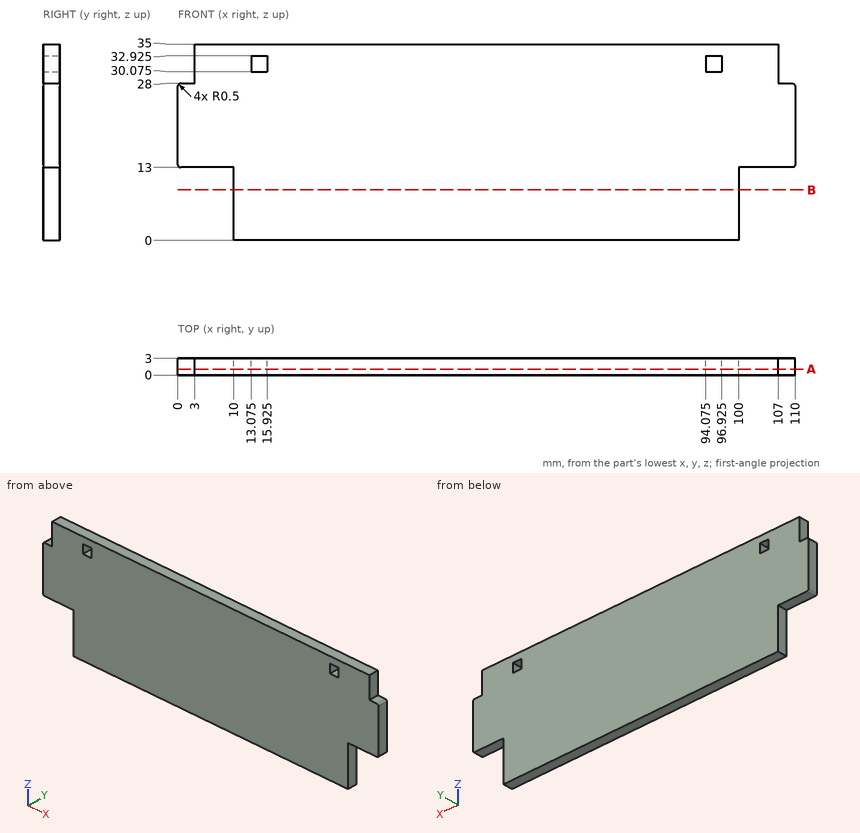
Study the drawing (mm; zero at the part's minimum x, y, z) and answer. Coordinates: 2 decimals unless noted, no trailing zeros. Write each loop counter-clockwise with the first axis right and the second up, starting at its lowest first coordinate (ties: lowest second). Pieces come first, ordered by that corner, then holes. Notation, with made-up numbers: (72.5, 64.25) -> (94.5, 64.25) arc R21 ccw to (94.5, 100.25) -> close; hole circle Ø5 at (9.5, 15). An arc over 180 degrees is marked (long way). Write item = value, one per line.
(1) Given pin 1 Ø0.9 at (y, z) = (1, 32.5) entering from +X; pin 2 Ø1.2 at (x, y) = (108.5, 1) entering from +Z; pin 3 Ø0.9 at (y, z) = (1, 32) entering from -X, each flat-ended and moving along its own axis, determine where each tip first touches the part or whether it passes through.
From the geometry:
pin_1 = 107
pin_2 = 28
pin_3 = 3
(2) Section A-A on y = 1.1 is taken. Write down the section's boundary in (x, z) (3 decimals).
From the geometry:
outline = (0, 13.5) arc R0.5 ccw to (0.5, 13) -> (10, 13) -> (10, 0) -> (100, 0) -> (100, 13) -> (109.5, 13) arc R0.5 ccw to (110, 13.5) -> (110, 27.5) arc R0.5 ccw to (109.5, 28) -> (107, 28) -> (107, 35) -> (3, 35) -> (3, 28) -> (0.5, 28) arc R0.5 ccw to (0, 27.5) -> close; hole (13.075, 30.075) -> (15.925, 30.075) -> (15.925, 32.925) -> (13.075, 32.925) -> close; hole (94.075, 30.075) -> (96.925, 30.075) -> (96.925, 32.925) -> (94.075, 32.925) -> close
(3) Straight lines are drawn through the part: L1, parallel to X at y = 2.6, z = 32 (3 decimals); L2, parallel to X at y = 1.3, z = 11; L3, parallel to Z at x = 102, y = 1.65. For each, find the intervals that lie inside material, in ascending order. Write a range as from..to.
From the geometry:
L1 = 3..13.075, 15.925..94.075, 96.925..107
L2 = 10..100
L3 = 13..35
(4) Section B-B on z = 9 is taken. Write down the section's boundary in (x, y).
From the geometry:
outline = (10, 0) -> (100, 0) -> (100, 3) -> (10, 3) -> close
